from build123d import *

# Parameters (mm, degrees)
F1_DEPTH = 3
F4_D     = 3
F6_D     = 3
F9_DEPTH = 34.3733802438


with BuildPart() as f1:
    # F0 (on Top) → F1 (new body)
    with BuildSketch(Plane.XY):
        Polygon((55, 0), (0, 0), (0, -143.1418224907), (20.0588525058, -143.1418224907), (85, -40), align=None)
        Polygon((20.0588525058, -143.1418224907), (0, -143.1418224907), (0, -175), align=None)
    extrude(amount=F1_DEPTH)

    # F4 (through all)
    with Locations(Plane.XY.offset(3)):
        with Locations((7.5, -130)):
            Hole(F4_D / 2)

    # F6 (through all)
    with Locations(Plane.XY.offset(3)):
        with Locations((31.7933925533, -30), (31.7933925533, -54), (31.7933925533, -5)):
            Hole(F6_D / 2)

    # F8 (on face) → F9 (cut)
    with BuildSketch(Plane.XY.offset(3)):
        with BuildLine():
            ThreePointArc((55.3, -17.5), (52.8, -15), (50.3, -17.5))
            Line((50.3, -17.5), (50.3, -62.5))
            ThreePointArc((50.3, -62.5), (52.8, -65), (55.3, -62.5))
            Line((55.3, -62.5), (55.3, -17.5))
        make_face()
    extrude(amount=-F9_DEPTH, mode=Mode.SUBTRACT)

    # F10: F1 across plane


with BuildPart() as f1_1:
    add(f1.part)
    add(f1.part.mirror(Plane.YZ))


solid = f1_1.part
Model file for the job. Use its own axes, mm. Give positions to 0.01 mm unless a question says otherwise; leave off trailing zeros. Order: outer loops, then holes, each group sorted by start corner. A loop starts at its lowest first (then second) coordinate and runs counter-clockwise, first axis right, second up. Notation, with made-up numbers: (4, 65.25) - (57, 65.25) arc R10 ccw to (57, 84.25) - close; hole circle Ø8 at (-40, 18.25). An arc over 180 degrees is marked (long way). Write item = value, one per line. Start each with the question number.
1. Cut at C-C, the plane x = 72. List the corners of the cut face in (y, z).
2. Cut at A-A, the plane z = 2. State how many separate pieces and enclosed holes the cut face has, and give its area (3 significant figures).
3. Cut at B-B, the plane x = 52.8. List the corners of the cut face in (y, z).
4. Cut at D-D, the plane x = -25. List the corners of the cut face in (y, z), and give its area (3 significant figures).
5. Probe line 1 along X through (y, z) = (-130, 1.2); line 2 along X through (y, z) = (-42, 2.85); line 3 along Y through (x, z) = (-7.5, 2.2). List the from-to ranges inside material, lowest first.
6. Drop flat-ended pins along their axis: P1, Ø1.8, axis at x = 31.79, y = -5, coming from the -Z side; P2, Ø5, axis at x = 31.79, y = -54, coming from the +Z side; P3, Ø1, axis at y = -25.5, z = 0.5, coming from the +X side; P4, Ø0.9, axis at y = -49.5, z = 1, coming from the -X side. Give the stop position or say it passes through.
Taken from the geometry:
q1.outline = (-60.65, 0) - (-22.67, 0) - (-22.67, 3) - (-60.65, 3) - close
q2.separate_pieces = 1
q2.enclosed_holes = 10
q2.area = 16,500 mm²
q3.outline = (-91.14, 0) - (-65, 0) - (-65, 3) - (-91.14, 3) - close; (-15, 0) - (0, 0) - (0, 3) - (-15, 3) - close
q4.outline = (-135.29, 0) - (0, 0) - (0, 3) - (-135.29, 3) - close
q4.area = 406 mm²
q5.line_1 = -28.33 to -9, -6 to 6, 9 to 28.33
q5.line_2 = -83.74 to -55.3, -50.3 to 50.3, 55.3 to 83.74
q5.line_3 = -163.09 to -131.5, -128.5 to 0
q6.P1 = through
q6.P2 = 3
q6.P3 = 74.5
q6.P4 = -79.3
